```python
from build123d import *

# Parameters (mm, degrees)
SKETCH1_W           = 14
SKETCH1_H           = 12
SKETCH1_W_2         = 60
SKETCH1_H_2         = 3
BOSS_EXTRUDE1_DEPTH = 15
CUT_EXTRUDE1_DEPTH  = 63.497999968


with BuildPart() as part:
    # Sketch1 → Boss-Extrude1 (new body)
    with BuildSketch(Plane(origin=(0, 0, 0), x_dir=(0, 0, -1), z_dir=(1, 0, 0))):
        with Locations((-7, 3)):
            Rectangle(SKETCH1_W, SKETCH1_H)
        with Locations((30, -1.5)):
            Rectangle(SKETCH1_W_2, SKETCH1_H_2)
    extrude(amount=-BOSS_EXTRUDE1_DEPTH)

    # Sketch6 → Cut-Extrude1 (cut, through all)
    with BuildSketch(Plane(origin=(0, 0, 0), x_dir=(0, 0, -1), z_dir=(1, 0, 0))):
        Polygon((0, 4.427403812), (0, 9), (-6.741112311, 9), (-11.084258062, 4.656854249), (-5.427403812, -1), align=None)
    extrude(amount=-CUT_EXTRUDE1_DEPTH, mode=Mode.SUBTRACT)


solid = part.part
```
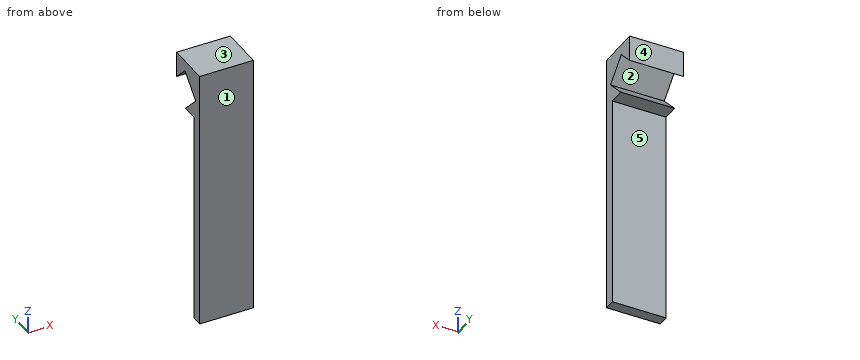
Geometry check sheet. Reference: the model listing, model coordinates, mm. Face numbers are marked on the shaded views. A direction names the side the tool comes from. Coordinates: 2 decimals unless noted, no trailing zeros. Order: outer loops, then holes, each group sorted by start corner. A loop starts at its lowest first (then second) coordinate and runs counter-clockwise, first axis right, second up. Notation, with made-up numbers: (1, 15) - (33, 15) arc R16 cw to (33, 45) - close; hole circle Ø10 at (50.25, -34.75). An arc over 180 degrees is marked (long way). Answer as a JSON object with one key per item and string values. Group by question number.
Item 1: Draft check along Z on the marked faces 1, 2 and 3. Enter one of: +Z half, -Z half, draft (parallel to the pull), parting line (faces both ways), or undercut.
Item 2: Tool access check on the marked faces 4 and 5. Record the directions out of +Z, -Z, +X, -X, +Y, -Y that give a thin tool (end or side, any length) a straight path to the whole face; none if there is none.
Item 3: Sectioned sample at A-A, the plane x = -9.75. Record the cut outline in (y, z), and give its area (3 significant figures).
Item 4: Scan lines: probe 1 along Z at (x, y) = (-14, 6.75); probe 2 along Y at (x, z) = (-11, -49.5); probe 3 along Z at (x, y) = (-0.75, 0.25). Record each from-to range of solid material in increasing order.
Item 5: Sectioned sample at D-D, the plane y = 5.5. Record the cut outline in (x, z), and give its area (3 significant figures).
Item 6: Sectioned sample at C-C, the plane z = -20. Record the cut outline in (x, y).
Item 7: Depth check by flat-ended pin: pin 1 Ø1 at (x, z) = (-10, -11) entering from +Y; pin 2 Ø2 at (x, y) = (-7, 1.5) entering from -Z; pin 3 Ø1 at (x, y) = (-4.5, 6) entering from -Z. Enter the tip coordinate at first touch or a pass-through.
Item 8: Sectioned sample at B-B, the plane y = 2. Record the cut outline in (x, z).
Resolved:
{
 "1": {"face 1": "draft", "face 2": "undercut", "face 3": "+Z half"},
 "2": {"face 4": "+Z, -Z, +X, -X, +Y", "face 5": "-Z, +X, -X, +Y"},
 "3": {"outline": "(-3, -60) - (0, -60) - (0, 0) - (4.43, 0) - (-1, 5.43) - (4.66, 11.08) - (9, 6.74) - (9, 14) - (-3, 14) - close", "area": "277 mm^2"},
 "4": {"probe 1": "8.99 to 14", "probe 2": "-3 to 0", "probe 3": "0 to 4.18, 6.68 to 14"},
 "5": {"outline": "(-15, 10.24) - (0, 10.24) - (0, 14) - (-15, 14) - close", "area": "56.4 mm^2"},
 "6": {"outline": "(-15, -3) - (0, -3) - (0, 0) - (-15, 0) - close"},
 "7": {"pin 1": "y = 0", "pin 2": "z = 0", "pin 3": "z = 9.24"},
 "8": {"outline": "(-15, 0) - (0, 0) - (0, 2.43) - (-15, 2.43) - close; (-15, 8.43) - (0, 8.43) - (0, 14) - (-15, 14) - close"}
}
